```python
from build123d import *

# Parameters (mm, degrees)
SKETCH_1_W          = 18
SKETCH_1_H          = 63.5
SKETCH_1_R          = 5
EXTRUDE_1_DEPTH     = 17
EXTRUDE_1_2_DEPTH   = 17
SKETCH_2_W          = 60
SKETCH_2_H          = 63.5
SKETCH_2_R          = 5
SKETCH_2_R_2        = 12
EXTRUDE_2_DEPTH     = 3
SKETCH_3_W          = 3
SKETCH_3_H          = 63.5
EXTRUDE_3_DEPTH     = 10
RIB_1_REACH         = 88.355
SKETCH_4_WALL_W     = 194.433823758
SKETCH_4_WALL_H     = 63.5
SKETCH_7_W          = 3
SKETCH_7_H          = 7
CUT_EXTRUDE_1_DEPTH = 3.5
HOLE_WIZARD_1_D     = 3.2
SKETCH_13_R         = 2.5
CUT_EXTRUDE_2_DEPTH = 11


with BuildPart() as part:
    # Sketch 1 → Extrude 1 (new body)
    with BuildSketch(Plane.XY):
        with Locations((36, 49.25)):
            Rectangle(SKETCH_1_W, SKETCH_1_H)
        with Locations((35, 49.25)):
            Circle(SKETCH_1_R, mode=Mode.SUBTRACT)
    extrude(amount=EXTRUDE_1_DEPTH)



with BuildPart() as body_2:
    # Sketch 1 → Extrude 1 2 (new body)
    with BuildSketch(Plane.XY):
        with Locations((-6, 49.25)):
            Rectangle(SKETCH_1_W, SKETCH_1_H)
        with Locations((-5, 49.25)):
            Circle(SKETCH_1_R, mode=Mode.SUBTRACT)
    extrude(amount=EXTRUDE_1_2_DEPTH)


with BuildPart() as part_1:
    add(part.part)

    add(body_2.part)  # Extrude 2 merges body 2
    # Sketch 2 → Extrude 2 (add)
    with BuildSketch(Plane.XY.offset(17)):
        with Locations((15, 49.25)):
            Rectangle(SKETCH_2_W, SKETCH_2_H)
        with Locations((35, 49.25)):
            Circle(SKETCH_2_R, mode=Mode.SUBTRACT)
        with Locations((-5, 49.25)):
            Circle(SKETCH_2_R, mode=Mode.SUBTRACT)
        with Locations((15, 49.25)):
            Circle(SKETCH_2_R_2, mode=Mode.SUBTRACT)
    extrude(amount=EXTRUDE_2_DEPTH)

    # Sketch 3 → Extrude 3 (add)
    with BuildSketch(Plane(origin=(45, 0, 0), x_dir=(0, 0, -1), z_dir=(1, 0, 0))):
        with Locations((-18.5, 49.25)):
            Rectangle(SKETCH_3_W, SKETCH_3_H)
    extrude(amount=EXTRUDE_3_DEPTH)

    # Sketch 4 wall → Rib 1 (add, up to next)
    with BuildSketch(Plane(origin=(50, 17.5, 8.5), x_dir=(-0.507020126563, 0, -0.861934215158), z_dir=(0.861934215158, 0, -0.507020126563)), mode=Mode.PRIVATE) as rib_1_sk1:
        with Locations((0, 31.75)):
            Rectangle(SKETCH_4_WALL_W, SKETCH_4_WALL_H)
    rib_1_tool1 = extrude(rib_1_sk1.sketch, amount=-RIB_1_REACH, mode=Mode.PRIVATE) - part_1.part
    add(rib_1_tool1.solids().sort_by_distance((50, 17.5, 8.5))[0])

    # Sketch 7 → Cut-Extrude 1 (cut, symmetric)
    with BuildSketch(Plane.XY.offset(10)):
        with Locations((-12.5, 49.25)):
            Rectangle(SKETCH_7_W, SKETCH_7_H)
        with Locations((42.5, 49.25)):
            Rectangle(SKETCH_7_W, SKETCH_7_H)
    extrude(amount=CUT_EXTRUDE_1_DEPTH, both=True, mode=Mode.SUBTRACT)

    # Hole Wizard 1 (through all)
    with Locations(Plane.ZY.offset(15)):
        with Locations((10, 49.25)):
            Hole(HOLE_WIZARD_1_D / 2)

    # Sketch 13 → Cut-Extrude 2 (cut)
    with BuildSketch(Plane.ZY.offset(-47)):
        with Locations((10, 49.25)):
            Circle(SKETCH_13_R)
    extrude(amount=-CUT_EXTRUDE_2_DEPTH, mode=Mode.SUBTRACT)


solid = part_1.part
```
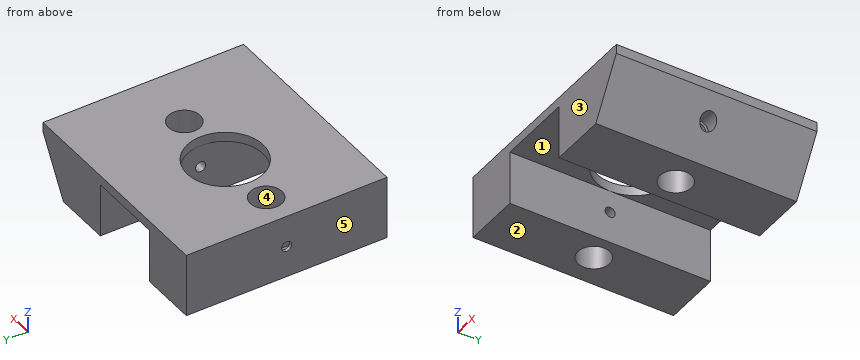
Source: CAD feature listing. Evaluate the final solid. Frame: model axes, mm. Face numbers are marked on the shaded views. A direction names the side the tool comes from. Give positions to 0.01 mm unless a question says otherwise; leave off trailing zeros. Loops run counter-clockwise (first coordinate to the right, second up) from the corner with the lowest first, then second, coordinate; pieces in that order, holes last. Notation, with made-up numbers: (6, 74.25) -> (54, 74.25) arc R21 ccw to (54, 92.25) -> close; hole circle Ø6 at (32.5, 16). An arc over 180 degrees is marked (long way). Put each result on its own line as item: value. Start each with the question number.
1) Cut plane C-C (y = 42). Return loops of the section in (x, z), then the cut area to 3 significant figures.
2) Cut plane A-A (x = 35). Return loops of the section in (y, z).
3) Cut plane B-B (z = 4.5). Return loops of the section in (x, y), then the cut area to 3 significant figures.
4) Reachability of the marked faces 1 and 2 from +Z, -Z, +X, -X, +Y, -Y: full face, straight path, thin tool, end or side. Return the list, or none.
5) Contact query for flat-ended pins moving along their axis: P1, Ø6, axis at x = 16, y = 74, coming from the -Z side; P2, Ø2, axis at y = 60, z = 13.5, coming from the +X side; P3, Ø5.5, axis at y = 48.5, z = 9.5, coming from the +X side. Output: stop coordinate, or through.
6) Material intervals for probe 1 along X at (y, z) = (60.5, 12.5); probe 2 along Z at (x, y) = (-10.7, 49.25); probe 3 along Y at (x, z) = (50.15, 10), sorted ascending.
7) Draft query along X for the marked faces 3, 4 and 5. Return one class per face: released by +X, released by -X, zero draft, split by the parting line, or undercut.
8) Cut plane D-D (y = 22.5). Return loops of the section in (x, z), then the cut area to 3 significant figures.
Results are:
1. outline: (-15, 0) -> (3, 0) -> (3, 17) -> (5.44, 17) -> (5.44, 20) -> (-15, 20) -> close; (24.56, 17) -> (27, 17) -> (27, 0) -> (45, 0) -> (55, 17) -> (55, 20) -> (24.56, 20) -> close
1. area: 850 mm2
2. outline: (17.5, 0) -> (44.25, 0) -> (44.25, 20) -> (17.5, 20) -> close; (54.25, 0) -> (81, 0) -> (81, 20) -> (54.25, 20) -> close
3. outline: (-15, 17.5) -> (3, 17.5) -> (3, 81) -> (-15, 81) -> close; (27, 17.5) -> (47.65, 17.5) -> (47.65, 81) -> (27, 81) -> close; hole circle Ø10 at (-5, 49.25); hole circle Ø10 at (35, 49.25)
3. area: 2,300 mm2
4. face 1: -Z, +Y, -Y
4. face 2: -Z, +X, -X, +Y, -Y
5. P1: stops at z = 17
5. P2: stops at x = 53.53
5. P3: stops at x = 52.19
6. probe 1: x = -15 to 3, 27 to 52.35
6. probe 2: z = 0 to 8.4, 11.6 to 20
6. probe 3: y = 17.5 to 46.75, 51.75 to 81
7. face 3: zero draft
7. face 4: undercut
7. face 5: released by -X
8. outline: (-15, 0) -> (3, 0) -> (3, 17) -> (27, 17) -> (27, 0) -> (45, 0) -> (55, 17) -> (55, 20) -> (-15, 20) -> close
8. area: 907 mm2
